from build123d import *

# Parameters (mm, degrees)
SKETCH1_W      = 12.9
SKETCH1_H      = 14.9
EXTRUDE1_DEPTH = 14.9
SKETCH2_W      = 9.8
SKETCH2_H      = 3.5
EXTRUDE2_DEPTH = 2.4
EXTRUDE3_DEPTH = 12.5
CHAMFER1_SIZE  = 1.2
CHAMFER1_SIZE2 = 3
FILLET1_R      = 0.2


with BuildPart() as part:
    # Sketch1 → Extrude1 (new body)
    with BuildSketch(Plane.XY):
        with Locations((6.45, 7.45)):
            Rectangle(SKETCH1_W, SKETCH1_H)
    extrude(amount=-EXTRUDE1_DEPTH)

    # Sketch2 → Extrude2 (cut)
    with BuildSketch(Plane.XY):
        with Locations((6.45, 13.15)):
            Rectangle(SKETCH2_W, SKETCH2_H)
    extrude(amount=-EXTRUDE2_DEPTH, mode=Mode.SUBTRACT)

    # Sketch3 → Extrude3 (cut)
    with BuildSketch(Plane.XY):
        Polygon((1.55, 11.4), (1.55, 3.1), (2.85, 3.1), (2.85, 2.1), (6.05, 2.1), (6.05, 3.1), (7.35, 3.1), (7.35, 4.8), (11.35, 4.8), (11.35, 11.4), align=None)
    extrude(amount=-EXTRUDE3_DEPTH, mode=Mode.SUBTRACT)

    # Chamfer1
    chamfer1_edges = [part.edges().sort_by_distance(p)[0] for p in [
        (4.45, 2.1, 0),
    ]]
    chamfer1_side = [part.faces().sort_by_distance(p)[0] for p in [
        (0.775, 14.702916261, 0),
    ]]
    chamfer(chamfer1_edges, length=CHAMFER1_SIZE, length2=CHAMFER1_SIZE2, reference=chamfer1_side[0])

    # Fillet1
    fillet1_edges = [part.edges().sort_by_distance(p)[0] for p in [
        (1.55, 13.15, -2.4),
        (6.45, 14.9, -2.4),
        (1.55, 14.9, -1.2),
        (11.35, 13.15, -2.4),
        (11.35, 14.9, -1.2),
        (6.45, 11.4, -2.4),
        (1.55, 9, 0),
        (11.35, 9.85, 0),
        (6.45, 11.4, -12.5),
        (1.55, 11.4, -7.45),
        (11.35, 8.1, -12.5),
        (11.35, 11.4, -7.45),
        (9.35, 4.8, -12.5),
        (7.35, 3.95, -12.5),
        (7.35, 4.8, -6.25),
        (6.7, 3.1, -12.5),
        (6.05, 2.6, -12.5),
        (6.05, 3.1, -6.25),
        (2.85, 2.6, -12.5),
        (2.2, 3.1, -12.5),
        (2.85, 3.1, -6.25),
        (1.55, 7.25, -12.5),
        (1.55, 3.1, -6.25),
        (2.2, 3.1, 0),
        (2.85, 1.5, 0),
        (6.05, 1.5, 0),
        (6.7, 3.1, 0),
        (7.35, 3.95, 0),
        (9.35, 4.8, 0),
    ]]
    fillet(fillet1_edges, radius=FILLET1_R)


solid = part.part
Can you work these out from the model? Positions are in its coordinate system, mm. A direction names the side the tool comes from. Coordinates: 2 decimals unless noted, no trailing zeros. Write each loop counter-clockwise with the first axis right and the second up, starting at its lowest first coordinate (ties: lowest second). Pieces come first, ordered by that corner, then holes. Notation, with made-up numbers: (78.25, 11.5) -> (83.25, 11.5) arc R31 ccw to (83.25, 36.5) -> close; hole circle Ø9 at (-23.5, -15). An arc over 180 degrees is marked (long way). Write item = value, one per line.
(1) Imagine slicing it at C-C (x = 8.75). Please give me the cut outline in (y, z), and give its area (3 significant figures).
Verdict:
outline = (0, -14.9) -> (14.9, -14.9) -> (14.9, -2.6) arc R0.2 ccw to (14.7, -2.4) -> (11.6, -2.4) arc R0.2 ccw to (11.4, -2.6) -> (11.4, -12.3) arc R0.2 cw to (11.2, -12.5) -> (5, -12.5) arc R0.2 cw to (4.8, -12.3) -> (4.8, -0.2) arc R0.2 ccw to (4.6, 0) -> (0, 0) -> close
area = 131 mm^2
(2) Imagine slicing it at D-D (z = -1.25). Please give me the cut outline in (x, y).
Verdict:
outline = (0, 0) -> (12.9, 0) -> (12.9, 14.9) -> (11.55, 14.9) arc R0.2 ccw to (11.35, 14.7) -> (11.35, 4.8) -> (7.55, 4.8) arc R0.2 ccw to (7.35, 4.6) -> (7.35, 3.1) -> (6.25, 3.1) arc R0.2 ccw to (6.05, 2.9) -> (6.05, 1.4) -> (2.85, 1.4) -> (2.85, 2.9) arc R0.2 ccw to (2.65, 3.1) -> (1.75, 3.1) arc R0.2 cw to (1.55, 3.3) -> (1.55, 14.7) arc R0.2 ccw to (1.35, 14.9) -> (0, 14.9) -> close
(3) Imagine slicing it at A-A (z = -8.75). Please give me the cut outline in (x, y).
Verdict:
outline = (0, 0) -> (12.9, 0) -> (12.9, 14.9) -> (0, 14.9) -> close; hole (1.55, 3.3) arc R0.2 ccw to (1.75, 3.1) -> (2.65, 3.1) arc R0.2 cw to (2.85, 2.9) -> (2.85, 2.1) -> (6.05, 2.1) -> (6.05, 2.9) arc R0.2 cw to (6.25, 3.1) -> (7.35, 3.1) -> (7.35, 4.6) arc R0.2 cw to (7.55, 4.8) -> (11.35, 4.8) -> (11.35, 11.2) arc R0.2 ccw to (11.15, 11.4) -> (1.75, 11.4) arc R0.2 ccw to (1.55, 11.2) -> close
(4) Imagine slicing it at B-B (y = 10.75). Please give me the cut outline in (x, z).
Verdict:
outline = (0, -14.9) -> (12.9, -14.9) -> (12.9, 0) -> (11.55, 0) arc R0.2 ccw to (11.35, -0.2) -> (11.35, -12.3) arc R0.2 cw to (11.15, -12.5) -> (1.75, -12.5) arc R0.2 cw to (1.55, -12.3) -> (1.55, -0.2) arc R0.2 ccw to (1.35, 0) -> (0, 0) -> close
(5) Thinking about a two-plate mould opening in X: for faces 1 (the face through (6, 13, -2.4)), 2 (the face through (6, 14.9, -9)), 3 (the face through (7, 3.1, -6)), 4 (the face through (12.9, 7, -7)), which applies, +X half, -X half, draft (parallel to the pull), parting line (faces both ways), or undercut?
Verdict:
face_1 = undercut
face_2 = draft
face_3 = undercut
face_4 = +X half
(6) For pin 1 (2.5 mm diameter, centred on x = 7, y = 7, fed in from +Z); pin 2 (1.6 mm diameter, centred on x = 8, y = 12.5, fed in from +Z); pin 3 (1 mm diameter, centred on x = 11, y = 7.5, fed in from +Z), each with a flat end and sliding along its axis, tell me the tip position at first contact or that it passes through.
Verdict:
pin_1 = -12.5
pin_2 = -2.4
pin_3 = -0.01
(7) On a 3-axis mill with a long thin cutter (end or side, diameter ignored), from which of +Z, -Z, +X, -X, +Y, -Y can I reach the whole of each face in a straight line? I mean faces 5 (the face through (0, 7, -7)), 6 (the face through (2.85, 2.4, -6.2)). Say none if no direction works.
Verdict:
face_5 = +Z, -Z, -X, +Y, -Y
face_6 = +Z
(8) If I drill on probe 1 along X at (y, z) = (7.5, -6); probe 2 along Y at (x, z) = (3, -12.25); probe 3 along Y at (x, z) = (7, -7), over which ranges is the centre line in solid material (lowest first)?
Verdict:
probe_1 = 0 to 1.55, 11.35 to 12.9
probe_2 = 0 to 2.1, 11.4 to 14.9
probe_3 = 0 to 3.1, 11.4 to 14.9
